Build history of the part. All positions in model axes, mm. A direction names the side the tool comes from. Round coordinates to 2 decimals unless told otherwise and drop trailing zeros. Write each loop counter-clockwise with the first axis right and the second up, starting at its lowest first coordinate (ties: lowest second). Pieces come first, ordered by that corner, then holes.
1) Which spindle directions (+Z, -Z, +X, -X, +Y, -Y) get a long thin tool onto all of the face, cutting with end or side? Do faces 1 (the flat face through (9, 86, 17.5)), 2 (the flat face through (19, 86, 9)). Say none if no direction does.
2) Wall check: probe 1 along Y at (x, z) = (9.5, 18.25); probe 2 along Z at (x, y) = (13.25, 148). Give the ranges that are in metal, low to high.
3) Saw through at C-C (y = 72.25). Write the cut outline in (x, z), plus the area to 3 significant figures.
4) Saw through at D-D (y = 39). Write the cut outline in (x, z), plus the area to 3 significant figures.
5) Pull direction Z, two halves, no side cores. Call faces 3 (the flat face through (1.5, 86, 9)), 4 (the flat face through (9, 89, 0)), 5 (the flat face through (9, 0, 18)): +Z half, -Z half, draft (parallel to the pull), parting line (faces both ways), or undercut.
6) Saw through at B-B (x = 9.5). Write the cut outline in (y, z), plus the area to 3 significant figures.
7) Saw through at A-A (z = 8). Write the cut outline in (x, y), plus the area to 3 significant figures.
Autodesk Inventor part; units mm, degrees
ref_plane "YZ Plane" through (0, 0, 0) normal (1, 0, 0) x (0, 1, 0)
ref_plane "XZ Plane" through (0, 0, 0) normal (0, 1, 0) x (-1, 0, 0)
ref_plane "XY Plane" through (0, 0, 0) normal (0, 0, 1) x (1, 0, 0)
sketch "Sketch1" plane through (0, 0, 0) normal (0, 0, 1) x (1, 0, 0)
  line L0 (0, 0) -> (19, 0)
  line L1 (19, 0) -> (19, 175)
  line L2 (19, 175) -> (0, 175)
  line L3 (0, 175) -> (0, 0)
  dimension "d0" = 19
  dimension "d1" = 175
extrude "Extrusion1" add sketch "Sketch1" along normal blind 19
sketch "Sketch2" plane through (0, 0, 0) normal (0, -1, 0) x (1, 0, 0)
  line L0 (0, 0) -> (19, 0)
  line L1 (19, 0) -> (19, 19)
  line L2 (0, 19) -> (19, 19)
  line L3 (0, 0) -> (0, 19)
  line L4 (17.5, 17.5) -> (17.5, 1.5)
  line L5 (17.5, 1.5) -> (1.5, 1.5)
  line L6 (1.5, 1.5) -> (1.5, 17.5)
  line L7 (1.5, 17.5) -> (17.5, 17.5)
  dimension "d4" = 1.5
extrude "Extrusion2" cut sketch "Sketch2" against normal through all contours L4 L5 L6 L7
sketch "Sketch3" plane through (0, 0, 19) normal (0, 0, 1) x (1, 0, 0)
  line L0 (9.5, 72.25) -> (9.5, 102.75) construction
  circle A0 centre (9.5, 102.75) radius 3
  circle A1 centre (9.5, 72.25) radius 4.5
  line L1 (19, 0) -> (19, 175)
  line L2 (19, 175) -> (0, 175)
  point P0 (0, 0)
  point P1 (19, 87.5)
  point P2 (9.5, 87.5)
  point P3 (9.5, 175)
  dimension "d7" = 30.5
  dimension "d8" = 6
  dimension "d9" = 9
extrude "Extrusion3" cut sketch "Sketch3" against normal through all
properties part number "C010" material "Aluminum 6061"
Evaluation:
1. face 1: +Y, -Y
1. face 2: +Z, -Z, +X, +Y, -Y
2. probe 1: y = 0 to 67.75, 76.75 to 99.75, 105.75 to 175
2. probe 2: z = 0 to 1.5, 17.5 to 19
3. outline: (0, 0) - (5, 0) - (5, 1.5) - (1.5, 1.5) - (1.5, 17.5) - (5, 17.5) - (5, 19) - (0, 19) - close; (14, 0) - (19, 0) - (19, 19) - (14, 19) - (14, 17.5) - (17.5, 17.5) - (17.5, 1.5) - (14, 1.5) - close
3. area: 78.0 mm2
4. outline: (0, 0) - (19, 0) - (19, 19) - (0, 19) - close; hole (1.5, 1.5) - (17.5, 1.5) - (17.5, 17.5) - (1.5, 17.5) - close
4. area: 105 mm2
5. face 3: undercut
5. face 4: -Z half
5. face 5: draft
6. outline: (0, 0) - (67.75, 0) - (67.75, 1.5) - (0, 1.5) - close; (0, 17.5) - (67.75, 17.5) - (67.75, 19) - (0, 19) - close; (76.75, 0) - (99.75, 0) - (99.75, 1.5) - (76.75, 1.5) - close; (76.75, 17.5) - (99.75, 17.5) - (99.75, 19) - (76.75, 19) - close; (105.75, 0) - (175, 0) - (175, 1.5) - (105.75, 1.5) - close; (105.75, 17.5) - (175, 17.5) - (175, 19) - (105.75, 19) - close
6. area: 480 mm2
7. outline: (0, 0) - (1.5, 0) - (1.5, 175) - (0, 175) - close; (17.5, 0) - (19, 0) - (19, 175) - (17.5, 175) - close
7. area: 525 mm2
